Geometry: final body of the model. Coordinates: model frame, mm. Face numbers are marked on the shaded views. A direction names the side the tool comes from. Coordinates: 2 decimals unless noted, no trailing zeros. Order: outer loops, then holes, each group sorted by start corner. A loop starts at its lowest first (then second) coordinate and runs counter-clockwise, first axis right, second up. Notation, with made-up numbers: M -20,48 L 20,48 A17 ccw 20,65 Z; hole C 66,11.25 d2. An arc over 180 degrees is marked long. Write item = value, one per line.
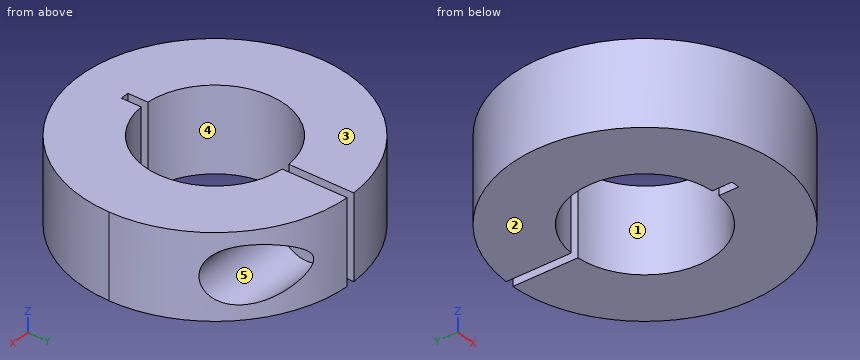
Autodesk Inventor part; units mm, degrees
ref_plane "Plan de construction1" through (4.25, 12.4775, 7.5) normal (1, 0, 0) x (0, 0, -1)
ref_plane "YZ Plane" through (0, 0, 0) normal (1, 0, 0) x (0, 1, 0)
ref_plane "XZ Plane" through (0, 0, 0) normal (0, 1, 0) x (-1, 0, 0)
sketch "Esquisse1" plane through (0, 0, 0) normal (0, 0, 1) x (1, 0, 0)
  circle A0 centre (0, 0) radius 12.5
  circle A1 centre (0, 0) radius 24
  dimension "d0" = 25
  dimension "d1" = 48
extrude "Extrusion1" add sketch "Esquisse1" along normal mid plane 15
sketch "Esquisse2" plane through (0, 0, 7.5) normal (0, 0, 1) x (1, 0, 0)
  line L0 (-0.75, 24) -> (0.75, 24)
  line L1 (0.75, 24) -> (0.75, -16)
  line L2 (0.75, -16) -> (-0.75, -16)
  line L3 (-0.75, -16) -> (-0.75, 24)
  line L4 (-0.75, 24) -> (0.75, -16) construction
  line L5 (0.75, 24) -> (-0.75, -16) construction
  circle A0 centre (0, 0) radius 24
  point P0 (0, 4)
  dimension "d4" = 1.5
  dimension "d5" = 40
extrude "Extrusion2" cut sketch "Esquisse2" against normal through all contours L0 A0 L3 | L0 L1 A0 | A0 L1 L2 L3 picked at (0, -2.6667)
ref_plane "Plan de construction1" through (4.25, 12.4775, 7.5) normal (1, 0, 0) x (0, 0, -1)
sketch "Esquisse3" plane through (4.25, 12.4775, 7.5) normal (1, 0, 0) x (0, 0, -1)
  line L0 (0, 11.5108) -> (15, 11.5108)
  line L1 (0, 0) -> (0, 11.5108)
  line L2 (15, 0) -> (0, 0)
  line L3 (15, 11.5108) -> (15, 0)
  point P0 (7.5, -12.4775)
  point P1 (7.4264, 5.4735)
hole "Perçage1" at (4.25, 17.951, 0.0736) direction (-1, 0, 0) diameter 4.134 depth 14 counterbore diameter 10 counterbore depth 2
sketch "Esquisse4" plane through (4.25, 12.4775, 7.5) normal (1, 0, 0) x (0, 0, -1)
  circle A0 centre (7.4264, 5.4735) radius 5
  point P0 (7.5, -12.4775)
extrude "Extrusion3" cut sketch "Esquisse4" along normal through all
properties part number "BagueSerrage"
1) Set-up query: the marked faces 3, 4 and 5. Return all of +Z, -Z, +X, -X, +Y, -Y with unobstructed straight access to the full face (end or side cutting, diameter ignored); none if empty.
Numbers:
face_3 = +Z, +X, -X, +Y, -Y
face_4 = +Z, -Z
face_5 = +X
2) Pin query (flat end, axial travel): pin 1 (4 mm diameter, centred on y = -4.5, z = -2.5, fed in from -X); pin 2 (4.5 mm diameter, centred on y = 18.5, z = 0, fed in from +X); pin 3 (3.5 mm diameter, centred on y = 17.95, z = 0.07, fed in from +X); pin 4 (12 mm diameter, centred on x = -2, y = -4.5, fed in from -Z) (3 decimals). Return the tip coordinate at first contact, or that it passes through.
Numbers:
pin_1 = -23.87
pin_2 = 2.25
pin_3 = -9.75
pin_4 = through
3) Section C-C, the plane z = 1. Return loops of the section in (x, y).
Numbers:
outline = M -9.75,16.1 L -9.75,19.8 L -0.75,19.8 L -0.75,23.99 A24 ccw long 20.15,13.04 L 2.25,13.04 L 2.25,16.1 L 0.75,16.1 L 0.75,12.48 A12.5 cw 0.75,-12.48 L 0.75,-16 L -0.75,-16 L -0.75,-12.48 A12.5 cw -0.75,12.48 L -0.75,16.1 Z; M 0.75,19.8 L 2.25,19.8 L 2.25,22.86 L 7.3,22.86 A24 ccw 0.75,23.99 Z
4) Section A-A, the plane x = -3. Return loops of the section in (y, z).
Numbers:
outline = M -23.81,-7.5 L -12.13,-7.5 L -12.13,7.5 L -23.81,7.5 Z; M 12.13,-7.5 L 23.81,-7.5 L 23.81,7.5 L 12.13,7.5 Z; hole C 17.95,0.07 d4.13
5) Section D-D, the plane y = -10.5. Return loops of the section in (x, z).
Numbers:
outline = M -21.58,-7.5 L -6.78,-7.5 L -6.78,7.5 L -21.58,7.5 Z; M 6.78,-7.5 L 21.58,-7.5 L 21.58,7.5 L 6.78,7.5 Z
6) Mould query, pull axis Y, two halves, no side actions, for the marked faces 1 and 2. Classes: pulls with the +Y half, pulls with the -Y half, needs draft (parallel to the pull), parting line crosses it, or undercut.
Numbers:
face_1 = undercut
face_2 = needs draft
7) Section B-B, the plane y = -1.5. Return loops of the section in (x, z).
Numbers:
outline = M -23.95,-7.5 L -12.41,-7.5 L -12.41,7.5 L -23.95,7.5 Z; M 12.41,-7.5 L 23.95,-7.5 L 23.95,7.5 L 12.41,7.5 Z
8) Line query: L1, parallel to Y at x = 10, z = 3.5; L2, parallel to Y at x = -0.5, z = 4; L3, parallel to X at y = -8.5, z = -6. Output: solid intervals per line, ascending.
Numbers:
L1 = -21.82 to -7.5, 7.5 to 14.31, 21.59 to 21.82
L2 = -23.99 to -16
L3 = -22.44 to -9.17, 9.17 to 22.44
